CAD build for the part. Positions are in the model's coordinates, mm. A direction names the side the tool comes from. Round coordinates to 2 decimals unless told otherwise and drop trailing zeros. Order: outer loops, then holes, each group sorted by start corner. A loop starts at its lowest first (then second) coordinate and runs counter-clockwise, first axis right, second up.
```python
from build123d import *

# Parameters (mm, degrees)
F0_W     = 76.2
F0_H     = 127
F0_W_2   = 25.4
F0_H_2   = 76.2
F1_DEPTH = 25.4
F2_T     = -2.54


with BuildPart() as f1:
    # F0 (on Front) → F1 (new body)
    with BuildSketch(Plane.XZ):
        with Locations((-38.1, 63.5)):
            Rectangle(F0_W, F0_H)
        with Locations((-38.1, 63.5)):
            Rectangle(F0_W_2, F0_H_2, mode=Mode.SUBTRACT)
    extrude(amount=F1_DEPTH)

    # F2
    f2_openings = [f1.faces().sort_by_distance(p)[0] for p in [
        (-38.1, -25.4, 1.481062),
    ]]
    offset(amount=F2_T, openings=f2_openings, kind=Kind.INTERSECTION)


solid = f1.part
```
1. Mould opens along X. For faces 4 (the face through (-76.2, -13, 63)), 5 (the face through (0, -13, 63)), 6 (the face through (-39, -13, 127)), 7 (the face through (-50.8, -13, 63)) say: released by +X, released by -X, zero draft, split by the parting line, or undercut.
2. Drill centre lines: line 1 (X direction, y = -6.75, z = 28); line 2 (Z direction, x = -24.5, y = -13.5); line 3 (Z direction, x = -33.5, y = -15). Where is each one in solid material? Low to high.
3. Pin check, flat tips, straight feed: P1, Ø11.5, axis at x = -38, y = -9, coming from the -Z side; P2, Ø5, axis at x = -32, z = 97.5, coming from the -Y side. Stop position of each tip, or through.
4. Cut at A-A, the plane x = -36. Write the cut outline in (y, z).
5. Cut at C-C, the plane z = 30. Write the cut outline in (x, y).
6. Tool access for faces 1 (the face through (-25.4, -13, 63)), 2 (the face through (-38, -14, 22.86)), 3 (the face through (-39, -13, 0)): list every direction of +Z, -Z, +X, -X, +Y, -Y with a clear straight run to the whole face (end or side of a thin tool).
7. Cut at B-B, the plane y = -8.5. Write the cut outline in (x, z).
8. Cut at D-D, the plane z = 115.5. Write the cut outline in (x, y), and give its area (3 significant figures).
Outcome:
1. face 4: released by -X
1. face 5: released by +X
1. face 6: zero draft
1. face 7: undercut
2. line 1: x = -76.2 to -73.66, -53.34 to -50.8, -25.4 to -22.86, -2.54 to 0
2. line 2: z = 0 to 2.54, 22.86 to 104.14, 124.46 to 127
2. line 3: z = 0 to 2.54, 22.86 to 25.4, 101.6 to 104.14, 124.46 to 127
3. P1: stops at z = 0
3. P2: passes through
4. outline: (-25.4, 0) - (0, 0) - (0, 25.4) - (-25.4, 25.4) - (-25.4, 22.86) - (-2.54, 22.86) - (-2.54, 2.54) - (-25.4, 2.54) - close; (-25.4, 101.6) - (0, 101.6) - (0, 127) - (-25.4, 127) - (-25.4, 124.46) - (-2.54, 124.46) - (-2.54, 104.14) - (-25.4, 104.14) - close
5. outline: (-76.2, -25.4) - (-73.66, -25.4) - (-73.66, -2.54) - (-53.34, -2.54) - (-53.34, -25.4) - (-50.8, -25.4) - (-50.8, 0) - (-76.2, 0) - close; (-25.4, -25.4) - (-22.86, -25.4) - (-22.86, -2.54) - (-2.54, -2.54) - (-2.54, -25.4) - (0, -25.4) - (0, 0) - (-25.4, 0) - close
6. face 1: +Y, -Y
6. face 2: -Y
6. face 3: -Z, +X, -X, +Y, -Y
7. outline: (-76.2, 0) - (0, 0) - (0, 127) - (-76.2, 127) - close; (-53.34, 22.86) - (-22.86, 22.86) - (-22.86, 104.14) - (-53.34, 104.14) - close; hole (-73.66, 2.54) - (-2.54, 2.54) - (-2.54, 124.46) - (-73.66, 124.46) - close; hole (-50.8, 25.4) - (-25.4, 25.4) - (-25.4, 101.6) - (-50.8, 101.6) - close
8. outline: (-76.2, -25.4) - (-73.66, -25.4) - (-73.66, -2.54) - (-2.54, -2.54) - (-2.54, -25.4) - (0, -25.4) - (0, 0) - (-76.2, 0) - close
8. area: 310 mm2
